from build123d import *

# Parameters (mm, degrees)
SKETCH1_W           = 20.5
SKETCH1_H           = 20.5
SKETCH1_R           = 62.5
BOSS_EXTRUDE1_DEPTH = 35
FILLET2_R           = 5
SKETCH2_W           = 20
SKETCH2_H           = 10
CUT_EXTRUDE2_DEPTH  = 7
SKETCH3_W           = 20
SKETCH3_H           = 10
CUT_EXTRUDE3_DEPTH  = 7


with BuildPart() as part:
    # Sketch1 → Boss-Extrude1 (new body)
    with BuildSketch(Plane.XY):
        with BuildLine():
            Line((117, -100.161277705), (117, -85.161277705))
            Line((117, -85.161277705), (88.226517383, -20.181680312))
            Line((88.226517383, -20.181680312), (108.734784021, -20.181680312))
            Line((108.734784021, -20.181680312), (108.734784021, 20.318319688))
            Line((108.734784021, 20.318319688), (69.594654141, 20.318319688))
            ThreePointArc((69.594654141, 20.318319688), (0, 72.5), (-69.594654141, 20.318319688))
            Line((-69.594654141, 20.318319688), (-108.734784021, 20.318319688))
            Line((-108.734784021, 20.318319688), (-108.734784021, -20.181680312))
            Line((-108.734784021, -20.181680312), (-88.226517383, -20.181680312))
            Line((-88.226517383, -20.181680312), (-117, -85.161277705))
            Line((-117, -85.161277705), (-117, -100.161277705))
            Line((-117, -100.161277705), (117, -100.161277705))
        make_face()
        with Locations((83.958397156, -79.911277705)):
            Rectangle(SKETCH1_W, SKETCH1_H, mode=Mode.SUBTRACT)
        with Locations((-83.958397156, -79.911277705)):
            Rectangle(SKETCH1_W, SKETCH1_H, mode=Mode.SUBTRACT)
        with BuildLine():
            Line((-63.708397156, -59.661277705), (-87.116280609, -59.661277705))
            Line((-87.116280609, -59.661277705), (-69.634400836, -20.181680312))
            ThreePointArc((-69.634400836, -20.181680312), (-46.29986484, -55.79043391), (-7, -72.161277705))
            Line((-7, -72.161277705), (-7, -85.161277705))
            Line((-7, -85.161277705), (-63.708397156, -85.161277705))
            Line((-63.708397156, -85.161277705), (-63.708397156, -59.661277705))
        make_face(mode=Mode.SUBTRACT)
        with BuildLine():
            Line((87.116280609, -59.661277705), (63.708397156, -59.661277705))
            Line((63.708397156, -59.661277705), (63.708397156, -85.161277705))
            Line((63.708397156, -85.161277705), (7, -85.161277705))
            Line((7, -85.161277705), (7, -72.161277705))
            ThreePointArc((7, -72.161277705), (46.29986484, -55.79043391), (69.634400836, -20.181680312))
            Line((69.634400836, -20.181680312), (87.116280609, -59.661277705))
        make_face(mode=Mode.SUBTRACT)
        with Locations((-88.484784021, 0.068319688)):
            Rectangle(SKETCH1_W, SKETCH1_H, mode=Mode.SUBTRACT)
        Circle(SKETCH1_R, mode=Mode.SUBTRACT)
        with Locations((88.484784021, 0.068319688)):
            Rectangle(SKETCH1_W, SKETCH1_H, mode=Mode.SUBTRACT)
    extrude(amount=BOSS_EXTRUDE1_DEPTH)

    # Fillet2
    fillet2_edges = [part.edges().sort_by_distance(p)[0] for p in [
        (-88.226517383, -20.181680312, 17.5),
        (-108.734784021, -20.181680312, 17.5),
        (-108.734784021, 20.318319688, 17.5),
        (-69.594654141, 20.318319688, 17.5),
        (69.594654141, 20.318319688, 17.5),
        (108.734784021, 20.318319688, 17.5),
        (108.734784021, -20.181680312, 17.5),
        (88.226517383, -20.181680312, 17.5),
        (7, -72.161277705, 17.5),
        (7, -85.161277705, 17.5),
        (63.708397156, -85.161277705, 17.5),
        (63.708397156, -59.661277705, 17.5),
        (-63.708397156, -59.661277705, 17.5),
        (-63.708397156, -85.161277705, 17.5),
        (-7, -85.161277705, 17.5),
        (-7, -72.161277705, 17.5),
    ]]
    fillet(fillet2_edges, radius=FILLET2_R)

    # Sketch2 → Cut-Extrude2 (cut)
    with BuildSketch(Plane(origin=(61.7, 0, 0), x_dir=(0, 0, -1), z_dir=(1, 0, 0))):
        with Locations((-17.5, 0.068319688)):
            Rectangle(SKETCH2_W, SKETCH2_H)
    extrude(amount=CUT_EXTRUDE2_DEPTH, mode=Mode.SUBTRACT)

    # Sketch3 → Cut-Extrude3 (cut)
    with BuildSketch(Plane(origin=(-61.7, 0, 0), x_dir=(0, 0, -1), z_dir=(1, 0, 0))):
        with Locations((-17.5, 0.068319688)):
            Rectangle(SKETCH3_W, SKETCH3_H)
    extrude(amount=-CUT_EXTRUDE3_DEPTH, mode=Mode.SUBTRACT)


solid = part.part
CAD build for the part. Positions are in the model's coordinates, mm. A direction names the side the tool comes from. Give positions to 0.01 mm unless a question says otherwise; leave off trailing zeros. Write each loop counter-clockwise with the first axis right and the second up, starting at its lowest first coordinate (ties: lowest second). Pieces come first, ordered by that corner, then holes. Notation, with made-up numbers: M 74,47.5 L 96,47.5 A12 ccw 96,54.5 Z; hole C 58,17 d5. An arc over 180 degrees is marked long. Put each result on its own line as item: value. Start each with the question number.
(1) Band-saw the part on B-B, the plane x = 0. Write the cut outline in (y, z).
(2) Which spindle directions (+Z, -Z, +X, -X, +Y, -Y) get a long thin tool onto all of the face, cutting with end or side? Do faces 4 (the face through (94.208, -80, 17)), 5 (the face through (91.681, -22.513, 17.745)), 6 (the face through (-65, 0, 7.5)). Say none if no direction does.
(3) Probe L1, parallel to Y at x = -90.5, z = 23.5; L2, parallel to X at y = 0, z = 13; L3, parallel to Y at x = 0, z = 9. List the from-to ranges inside material, lowest first.
(4) Band-saw the part on A-A, the plane y = 0. Write the cut outline in (x, z), and give its area (3 significant figures).
(5) Band-saw the part on D-D, the plane y = 58. Write the cut outline in (x, z), and give its area (3 significant figures).
(6) Band-saw the part on C-C, the plane x = -45. Write the cut outline in (y, z).
(7) Flat gauge pins, fed straight in: pin 1 Ø6 at (y, z) = (-4.5, 23.5) entering from -X; pin 2 Ø10.5 at (x, z) = (-25, 10) entering from +Y; pin 3 Ø10 at (x, z) = (-91.5, 13.5) entering from +Y; pin 4 Ø3 at (x, y) = (-66, 2.5) entering from -Z. Where does each tip first touch, or does it go through?
(8) Mould opens along Z. For faces 1 (the face through (63.708, -72, 17)), 2 (the face through (-65, -4.932, 18)), 3 (the face through (-65, 5.068, 18)) say: +Z half, -Z half, draft (parallel to the pull), parting line (faces both ways), or undercut.
Response values:
1. outline: M -100.16,0 L -62.5,0 L -62.5,35 L -100.16,35 Z; M 62.5,0 L 72.5,0 L 72.5,35 L 62.5,35 Z
2. face 4: +Z, -Z
2. face 5: +Z, -Z, +X
2. face 6: none
3. L1: y = -100.16 to -90.16, -69.66 to -10.18, 10.32 to 20.32
3. L2: x = -108.73 to -98.73, -78.23 to -68.7, 68.7 to 78.23, 98.73 to 108.73
3. L3: y = -100.16 to -62.5, 62.5 to 72.5
4. outline: M -108.73,0 L -98.73,0 L -98.73,35 L -108.73,35 Z; M -78.23,0 L -62.5,0 L -62.5,7.5 L -68.7,7.5 L -68.7,27.5 L -62.5,27.5 L -62.5,35 L -78.23,35 Z; M 62.5,0 L 78.23,0 L 78.23,35 L 62.5,35 L 62.5,27.5 L 68.7,27.5 L 68.7,7.5 L 62.5,7.5 Z; M 98.73,0 L 108.73,0 L 108.73,35 L 98.73,35 Z
4. area: 1,550 mm2
5. outline: M -43.5,0 L -23.29,0 L -23.29,35 L -43.5,35 Z; M 23.29,0 L 43.5,0 L 43.5,35 L 23.29,35 Z
5. area: 1,410 mm2
6. outline: M -100.16,0 L -85.16,0 L -85.16,35 L -100.16,35 Z; M -56.84,0 L -43.37,0 L -43.37,35 L -56.84,35 Z; M 43.37,0 L 56.84,0 L 56.84,35 L 43.37,35 Z
7. pin 1: stops at x = -108.73
7. pin 2: stops at y = 69.76
7. pin 3: stops at y = 20.32
7. pin 4: stops at z = 0
8. face 1: draft
8. face 2: undercut
8. face 3: undercut
